Geometry check sheet. Reference: the model listing, model coordinates, mm. A direction names the side the tool comes from. Coordinates: 2 decimals unless noted, no trailing zeros. Write each loop counter-clockwise with the first axis right and the second up, starting at its lowest first coordinate (ties: lowest second). Pieces come first, ordered by that corner, then holes. Notation, with made-up numbers: (7.25, 13.5) -> (49.25, 13.5) arc R24 ccw to (49.25, 37.5) -> close; hole circle Ø6 at (48.5, 0.5). An arc over 180 degrees is marked (long way). Answer as CSV lines item,"result".
Autodesk Inventor part; units mm, degrees
ref_plane "Plano de trabajo1" through (0, 0, 0) normal (1, 0, 0) x (0, 0, -1)
ref_plane "YZ Plane" through (0, 0, 0) normal (1, 0, 0) x (0, 1, 0)
ref_plane "XZ Plane" through (0, 0, 0) normal (0, 1, 0) x (-1, 0, 0)
sketch "Boceto1" plane through (0, 0, 0) normal (0, 1, 0) x (-1, 0, 0)
  line L0 (0, 0) -> (35, 0)
  line L1 (47.5, -12.5) -> (47.5, -12.5)
  line L2 (35, -25) -> (0, -25)
  line L3 (0, -25) -> (0, 0)
  line L4 (47.5, -12.5) -> (0, -12.5) construction
  arc A0 (47.5, -12.5) -> (35, 0) centre (35, -12.5) ccw
  arc A1 (35, -25) -> (47.5, -12.5) centre (35, -12.5) ccw
  circle A2 centre (35, -12.5) radius 5
  point P0 (47.5, -25)
  point P1 (47.5, 0)
  dimension "d0" = 25
  dimension "d1" = 47.5
  dimension "d15" = 12.5
  dimension "d16" = 10
ref_plane "Plano de trabajo1" through (0, 0, 0) normal (1, 0, 0) x (0, 0, -1)
extrude "Extrusión3" add sketch "Boceto1" along normal blind 25
sketch "Boceto3" plane through (0, 0, 0) normal (1, 0, 0) x (0, 0, -1)
  circle A0 centre (12.5, 12.5) radius 5
  line L0 (25, 0) -> (25, 25)
  line L1 (0, 25) -> (25, 25)
  point P0 (0, 0)
  dimension "d19" = 10
  dimension "d20" = 12.5
  dimension "d21" = 12.5
extrude "Extrusión4" add sketch "Boceto3" along normal blind 20
thread "Rosca3"
thread "Rosca4"
properties part number "brazos_planetarios1" material "Acetal Resin, Black"
Item 1: Cross-section at D-D, the plane y = 22. Record the cut outline in (x, z), plus the area to 3 significant figures.
Responses:
outline,"(-35, -25) -> (0, -25) -> (0, 0) -> (-35, 0) arc R12.5 ccw to start; hole circle Ø10 at (-35, -12.5)"
area,"1,040 mm2"
Item 2: Set-up check for faces 1 (the flat face through (-23, 25, -12)), 2 (the cylindrical face through (9.86, 11, -17.27)): record each of +Z, -Z, +X, -X, +Y, -Y from which the full face is reachable in a straight line by a thin tool's end or side.
Responses:
face 1,"+Z, -Z, +X, -X, +Y"
face 2,"+X"
Item 3: Cross-section at C-C, the plane x = 9. Record the cut outline in (y, z).
Responses:
outline,"circle Ø10 at (12.5, -12.5)"
Item 4: Cross-section at B-B, the plane y = 11. Record the cut outline in (x, z), plus the area to 3 significant figures.
Responses:
outline,"(-35, -25) -> (0, -25) -> (0, -17.27) -> (20, -17.27) -> (20, -7.73) -> (0, -7.73) -> (0, 0) -> (-35, 0) arc R12.5 ccw to start; hole circle Ø10 at (-35, -12.5)"
area,"1,230 mm2"
Item 5: Cross-section at A-A, the plane z = -12.5. Record the cut outline in (x, y).
Responses:
outline,"(-47.5, 0) -> (-40, 0) -> (-40, 25) -> (-47.5, 25) -> close; (-30, 0) -> (0, 0) -> (0, 7.5) -> (20, 7.5) -> (20, 17.5) -> (0, 17.5) -> (0, 25) -> (-30, 25) -> close"
Item 6: Depth check by flat-ended pin: pin 1 Ø3 at (y, z) = (4.5, -16.5) entering from +X; pin 2 Ø3 at (y, z) = (6, -14.5) entering from -X; pin 3 Ø6 at (x, z) = (-35, -12.5) entering from +Y; pin 4 Ø8 at (x, z) = (9, -15.5) entering from -Y. Enter the tip coordinate at first touch or a pass-through.
Responses:
pin 1,"stops at x = 0"
pin 2,"stops at x = -47.49"
pin 3,"passes through"
pin 4,"stops at y = 7.5"
Item 7: Release check for a two-part mould opening along Z. For faces 3 (the flat face through (20, 13, -12)), 4 (the cylindrical face through (-30.005, 12.325, -12.72)), 5 (the cylindrical face through (-47.497, 12.325, -12.225)) record: +Z half, -Z half, draft (parallel to the pull), parting line (faces both ways), or undercut.
Responses:
face 3,"draft"
face 4,"undercut"
face 5,"parting line"
Item 8: Thickness scan on probe 1 along Z at (x, y) = (-35, 15.25); probe 2 along X at (y, z) = (19.75, -10.75); probe 3 along X at (y, z) = (17, -9.75). Record the ranges inside material, lowest first.
Responses:
probe 1,"z = -25 to -17.5, -7.5 to 0"
probe 2,"x = -47.38 to -39.68, -30.32 to 0"
probe 3,"x = -47.19 to -39.18, -30.82 to 0"
